Print and shaded views of the part. All mm, measured from the part's lowest x, y and z. A direction names the side the tool comes from. Coordinates: 2 decimals unless noted, no trailing zeros. Order: outer loops, then holes, each group sorted by start corner. A loop starts at its lowest first (then second) coordinate and runs counter-clockwise, first axis right, second up. Notation, with made-up numbers: (15, -2) -> (46, -2) arc R18 ccw to (46, 23) -> close; hole circle Ø5 at (-22, -16.5). An arc over 180 degrees is marked (long way). Return JSON: item names as keys, results as strings. Group by question number.
1) Cut at A-A (y = 12.5). Write the cut outline in (x, z) (3 decimals), and give its area (3 significant figures).
2) Probe line 1 (Y direction, x = 12.5, z = 5.25); line 2 (Y direction, x = 12.5, z = 9.25) (3 decimals); line 3 (Z direction, x = 13.5, y = 15.75). List the from-to ranges inside material, lowest first.
3) Flat gauge pins, fed straight in: pin 1 (12.5 mm diameter, centred on x = 12.5, y = 12.5, fed in from +Z); pin 2 (3 mm diameter, centred on x = 10, y = 12.5, fed in from +Z). Where does each tip first touch, or does it go through?
4) Cut at C-C (z = 2). Write the cut outline in (x, y).
5) Pull direction X, two halves, no side cores. Call the marked faces 3, 4 and 5: +X half, -X half, draft (parallel to the pull), parting line (faces both ways), or undercut.
6) Which spindle directions (+Z, -Z, +X, -X, +Y, -Y) get a long thin tool onto all of the face, cutting with end or side? Do the marked faces 1 and 2. Say none if no direction does.
7) Cut at D-D (x = 18). Write the cut outline in (y, z).
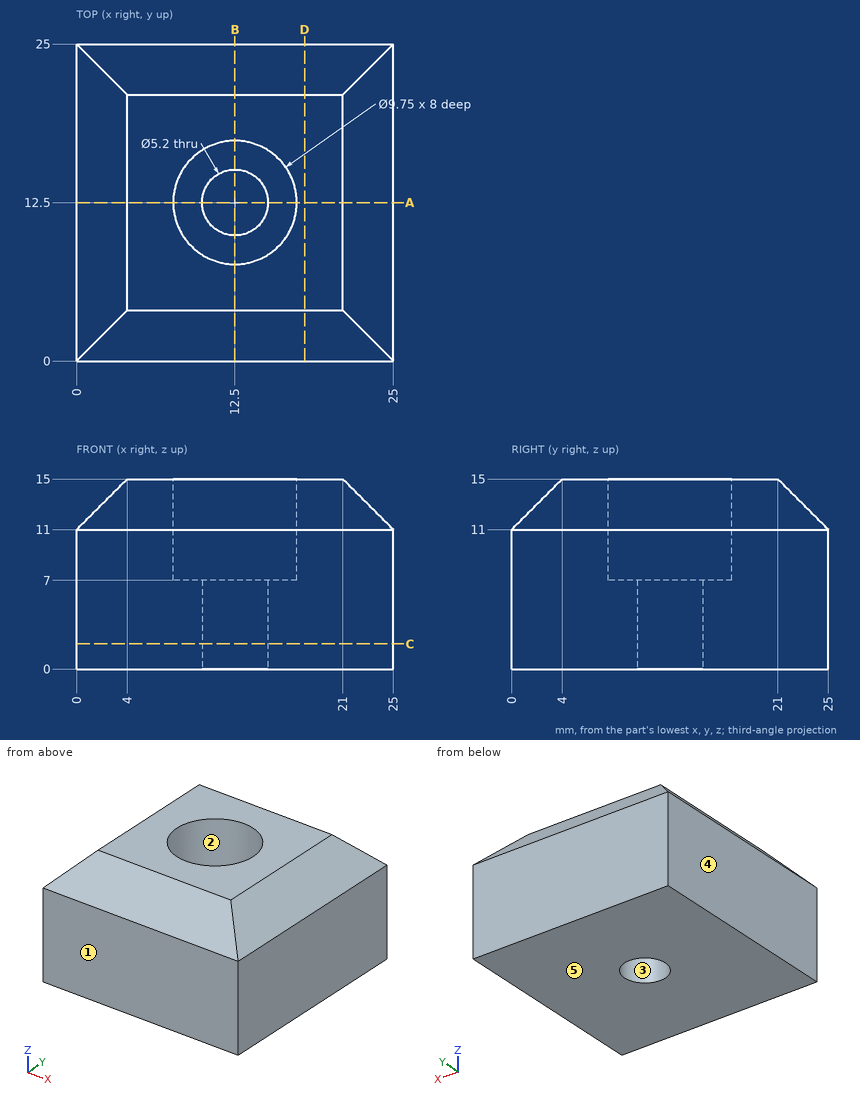
Answers below:
{
 "1": {"outline": "(0, 0) -> (9.9, 0) -> (9.9, 7) -> (7.625, 7) -> (7.625, 15) -> (4, 15) -> (0, 11) -> close; (15.1, 0) -> (25, 0) -> (25, 11) -> (21, 15) -> (17.375, 15) -> (17.375, 7) -> (15.1, 7) -> close", "area": "245 mm^2"},
 "2": {"line 1": "y = 0 to 9.9, 15.1 to 25", "line 2": "y = 0 to 7.625, 17.375 to 25", "line 3": "z = 0 to 7"},
 "3": {"pin 1": "stops at z = 15", "pin 2": "stops at z = 7"},
 "4": {"outline": "(0, 0) -> (25, 0) -> (25, 25) -> (0, 25) -> close; hole circle Ø5.2 at (12.5, 12.5)"},
 "5": {"face 3": "undercut", "face 4": "-X half", "face 5": "draft"},
 "6": {"face 1": "+Z, -Z, +X, -X, -Y", "face 2": "+Z"},
 "7": {"outline": "(0, 0) -> (25, 0) -> (25, 11) -> (21, 15) -> (4, 15) -> (0, 11) -> close"}
}
